Read the model definition and answer for the solid it produces. Units are mm, in the model's axes. Face numbers are marked on the shaded views. A direction names the side the tool comes from. Coordinates: 2 decimals unless noted, no trailing zeros. Loops run counter-clockwise (first coordinate to the right, second up) from the corner with the lowest first, then second, coordinate; pieces in that order, holes last. Notation, with made-up numbers: (23.5, -23) - (59.5, -23) arc R24 cw to (59.5, -3) - close; hole circle Ø1 at (25.25, -10). An arc over 180 degrees is marked (long way). Use CSV: the item, a comma, the result in double quotes.
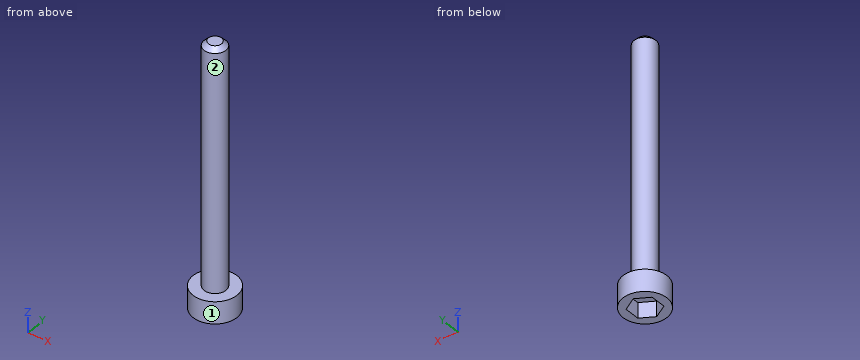
Solid Edge part; units mm, degrees
sketch "Sketch1" plane through (0, 0, 0) normal (0, 0, 1) x (1, 0, 0)
  circle A0 centre (0, 0) radius 10
extrude "Protrusion1" add sketch "Sketch1" along normal blind 10
sketch "Sketch2" plane through (0, 0, 10) normal (0, 0, 1) x (1, 0, 0)
  circle A0 centre (0, 0) radius 5
extrude "ExtrudedProtrusion_2" add sketch "Sketch2" along normal blind 110
cosmetic_thread "Thread_2" thread depth 15
chamfer "Chamfer_1" distance 2 angle 45 1 edges at (-5, 0, 120)
sketch "Sketch3" plane through (0, 0, 0) normal (0, 0, -1) x (0, 1, 0)
  line L0 (-3.4641, 6) -> (-6.9282, 0)
  line L1 (-6.9282, 0) -> (-3.4641, -6)
  line L2 (-3.4641, -6) -> (3.4641, -6)
  line L3 (3.4641, -6) -> (6.9282, 0)
  line L4 (6.9282, 0) -> (3.4641, 6)
  line L5 (3.4641, 6) -> (-3.4641, 6)
extrude "ExtrudedCutout_1" cut sketch "Sketch3" against normal blind 7
properties part number "1002"
Q1. A tool of negligible diameter and unlimited length cuts with its end or side. For the marked faces 1 and 2, from which of +Z, -Z, +X, -X, +Y, -Y can it reach the whole face along a straight path? Write none if from no direction.
Reported:
face 1,"+Z, -Z"
face 2,"+Z"
Q2. Given P1, Ø3.5, axis at x = 1.5, y = 0, coming from the -Z side; P2, Ø10, axis at y = -5.5, z = 105, coming from the -X side; P3, Ø8, axis at x = -5, z = 28, coming from the -Y side; P4, Ø4, axis at x = 8, z = 28, coming from the -Y side, each flat-ended and moving along its own axis, determine where each tip first touches the part or whether it passes through.
Reported:
P1,"stops at z = 7"
P2,"stops at x = -4.97"
P3,"stops at y = -4.9"
P4,"passes through"
Q3. The part is cut by section B-B on z = 102. Determine the outline of the cut face in (x, y), and give its area (3 significant figures).
Reported:
outline,"circle Ø10 at (0, 0)"
area,"78.5 mm²"
Q4. The part is cut by section D-D on y = 8. Determine the outline of the cut face in (x, z), and give its area (3 significant figures).
Reported:
outline,"(-6, 0) - (6, 0) - (6, 10) - (-6, 10) - close"
area,"120 mm²"
Q5. The part is cut by section C-C on x = 7. Determine the outline of the cut face in (y, z).
Reported:
outline,"(-7.14, 0) - (7.14, 0) - (7.14, 10) - (-7.14, 10) - close"
Q6. Find the intervals of material crossed by probe 1 along Z at (x, y) = (7.25, -2.25); probe 2 along Y at (x, z) = (-0.5, 13.5); probe 3 along Z at (x, y) = (0.5, -0.75), in increasing order. Write a range as [from, to].
Reported:
probe 1,"z = [0, 10]"
probe 2,"y = [-4.97, 4.97]"
probe 3,"z = [7, 120]"
Q7. The part is cut by section A-A on y = 0. Determine the outline of the cut face in (x, z), and give its area (3 significant figures).
Reported:
outline,"(-10, 0) - (-6, 0) - (-6, 7) - (6, 7) - (6, 0) - (10, 0) - (10, 10) - (5, 10) - (5, 118) - (3, 120) - (-3, 120) - (-5, 118) - (-5, 10) - (-10, 10) - close"
area,"1,210 mm²"
